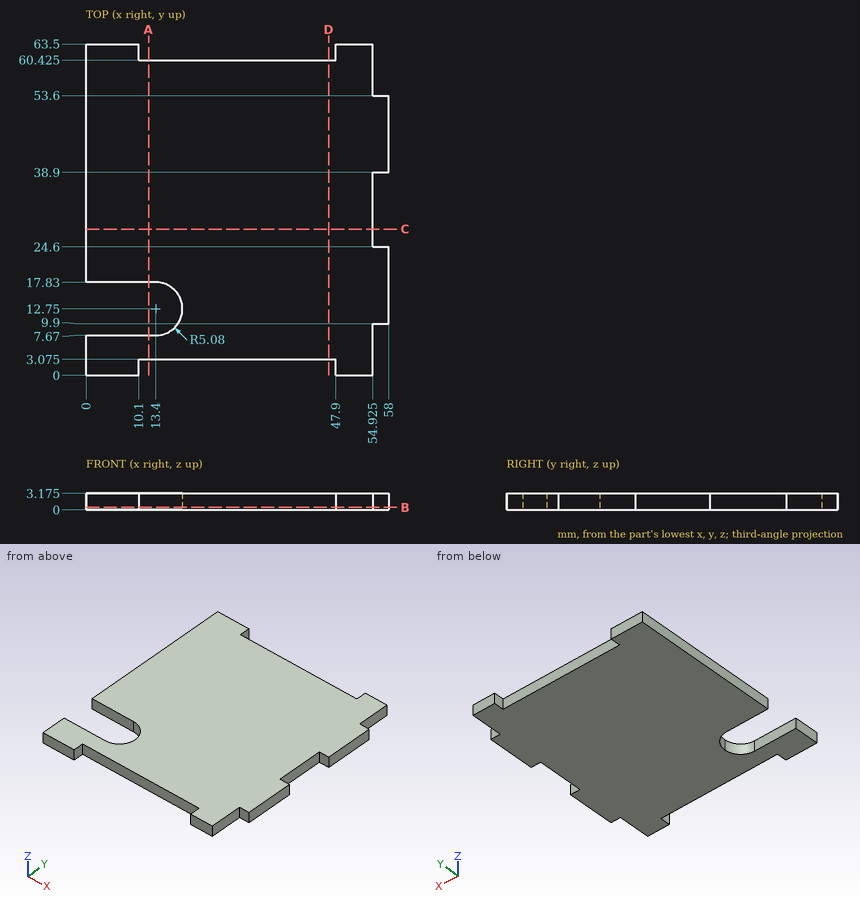
Source: three-view drawing plus pictorial views. Frame: mm from the lowest corner of the part. Round coordinates to 2 decimals unless told otherwise and drop trailing zeros. Loops run counter-clockwise (first coordinate to the right, second up) from the corner with the lowest first, then second, coordinate; pieces in that order, holes last. Notation, with made-up numbers: M 8,81 L 15,81 A16 ccw 15,92 Z; hole C 23.5,40 d8. An arc over 180 degrees is marked long. Put each result on its own line as item: value.
(1) First-contact query: pin 1 (0.9 mm diameter, centred on x = 56, z = 2, fed in from -Y); pin 2 (1.5 mm diameter, centred on x = 56, z = 1.5, fed in from +Y); pin 3 (0.9 mm diameter, centred on y = 1.5, z = 1, fed in from +X) (3 decimals). Flat tips, straight axial feed; report the tip coordinate or a pass-through.
Solutions:
pin 1: y = 9.9
pin 2: y = 53.6
pin 3: x = 54.925
(2) Ray query, line 1 (Y direction, x = 4.5, z = 1.25); line 2 (Y direction, x = 13, z = 0.7) (3 decimals); line 3 (Y direction, x = 35, z = 0.95) (3 decimals). Return the intervals inside material, ascending. Write a range as [from, to].
Solutions:
line 1: [0, 7.67], [17.83, 63.5]
line 2: [3.075, 7.67], [17.83, 60.425]
line 3: [3.075, 60.425]
(3) Section C-C, the plane y = 28. Return loops of the section in (x, z) (3 decimals), and give its area (3 significant figures).
Solutions:
outline: M 0,0 L 54.925,0 L 54.925,3.175 L 0,3.175 Z
area: 174 mm²
(4) Section B-B, the plane z = 0.5. Return loops of the section in (x, y) (3 decimals), and give its area (3 significant figures).
Solutions:
outline: M 0,0 L 10.1,0 L 10.1,3.075 L 47.9,3.075 L 47.9,0 L 54.925,0 L 54.925,9.9 L 58,9.9 L 58,24.6 L 54.925,24.6 L 54.925,38.9 L 58,38.9 L 58,53.6 L 54.925,53.6 L 54.925,63.5 L 47.9,63.5 L 47.9,60.425 L 10.1,60.425 L 10.1,63.5 L 0,63.5 L 0,17.83 L 13.4,17.83 A5.08 cw 13.4,7.67 L 0,7.67 Z
area: 3,170 mm²
(5) Section D-D, the plane x = 46.5. Return loops of the section in (y, z) (3 decimals), and give its area (3 significant figures).
Solutions:
outline: M 3.075,0 L 60.425,0 L 60.425,3.175 L 3.075,3.175 Z
area: 182 mm²
(6) Section A-A, the plane x = 12. Return loops of the section in (y, z) (3 decimals).
Solutions:
outline: M 3.075,0 L 7.67,0 L 7.67,3.175 L 3.075,3.175 Z; M 17.83,0 L 60.425,0 L 60.425,3.175 L 17.83,3.175 Z
